Here's how the part is built. I have some questions about the finished solid (model axes, mm). Face numbers are marked on the shaded views. A direction names the side the tool comes from. Give positions to 0.01 mm unless a question says otherwise; leave off trailing zeros. Loops run counter-clockwise (first coordinate to the right, second up) from the corner with the lowest first, then second, coordinate; pieces in that order, holes last. Notation, with made-up numbers: (-17.5, -22) - (19.5, -22) arc R34 cw to (19.5, 15) - close; hole circle Ø6 at (-30.75, 48). An arc over 180 degrees is marked (long way). Use a Markdown table: item, result.
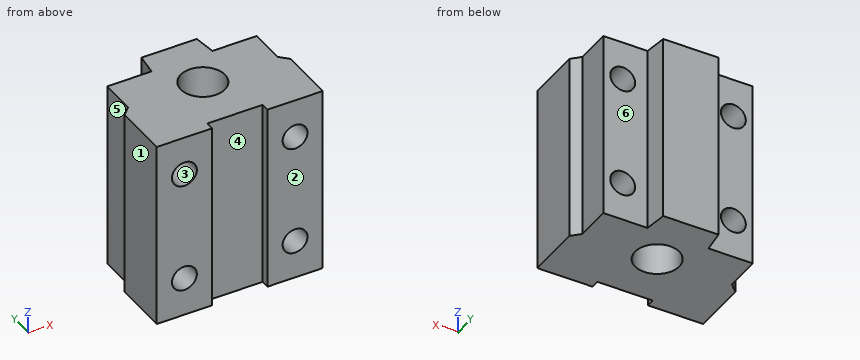
from build123d import *

# Parameters (mm, degrees)
SKETCH1_R           = 4
BOSS_EXTRUDE1_DEPTH = 34
SKETCH2_R           = 2.25
CUT_EXTRUDE1_DEPTH  = 42.291645644


with BuildPart() as part:
    # Sketch1 → Boss-Extrude1 (new body)
    with BuildSketch(Plane.XY):
        Polygon((5, -10), (-5, -10), (-5, -11.5), (-15, -11.5), (-15, -1.5), (-13.5, 0), (-13.5, 6.5), (-5.5, 6.5), (-5, 10.5), (5, 10.5), (5.5, 6.5), (13.5, 6.5), (13.5, 0), (15, -1.5), (15, -11.5), (5, -11.5), align=None)
        Circle(SKETCH1_R, mode=Mode.SUBTRACT)
    extrude(amount=BOSS_EXTRUDE1_DEPTH)

    # Sketch2 → Cut-Extrude1 (cut, through all)
    with BuildSketch(Plane(origin=(0, 6.5, 0), x_dir=(1, 0, 0), z_dir=(0, 1, 0))):
        with Locations(Location((10, -27, 0), (0, 0, 270))):
            Circle(SKETCH2_R)
        with Locations(Location((10, -7, 0), (0, 0, 270))):
            Circle(SKETCH2_R)
    cut_extrude1 = extrude(amount=-CUT_EXTRUDE1_DEPTH, mode=Mode.SUBTRACT)

    # Mirror1: Cut-Extrude1 across plane
    add(cut_extrude1.mirror(Plane(origin=(0, 0, 0), x_dir=(0, 0, 1), z_dir=(1, 0, 0))), mode=Mode.SUBTRACT)


solid = part.part
(1) Suppose I cut it at B-B on x = 0. Write out the boundary of the cut face in (y, z), plus the area to 3 significant figures.
A:
| item | result |
|---|---|
| outline | (-10, 0) - (-4, 0) - (-4, 34) - (-10, 34) - close; (4, 0) - (10.5, 0) - (10.5, 34) - (4, 34) - close |
| area | 425 mm2 |
(2) We'd pull the mould along X, two halves only. Please class the marked faces 1, 2 and 3: pulls with the +X half, pulls with the -X half, needs draft (parallel to the pull), parting line crosses it, or undercut.
A:
| item | result |
|---|---|
| face 1 | pulls with the -X half |
| face 2 | needs draft |
| face 3 | undercut |
(3) On a 3-axis mill with a long thin cutter (end or side, diameter ignored), from which of +Z, -Z, +X, -X, +Y, -Y can I reach the whole of each face in a straight line? I mean the marked faces 4, 5 and 6. Say none if no direction works.
A:
| item | result |
|---|---|
| face 4 | +Z, -Z, -Y |
| face 5 | +Z, -Z, -X, +Y |
| face 6 | +Z, -Z, +X, +Y |
(4) If I drill on line 1 (Z direction, x = -10, y = -3); line 2 (X direction, y = 0.25, z = 7); line 3 (X direction, y = -5.25, z = 27), over which ranges is the centre line in solid material (lowest first)?
A:
| item | result |
|---|---|
| line 1 | 0 to 4.75, 9.25 to 24.75, 29.25 to 34 |
| line 2 | -13.5 to -12.25, -7.75 to -3.99, 3.99 to 7.75, 12.25 to 13.5 |
| line 3 | -15 to -12.25, -7.75 to 7.75, 12.25 to 15 |
(5) Suppose I cut it at D-D on x = -10. Write out the boundary of the cut face in (y, z), plus the area to 3 significant figures.
A:
| item | result |
|---|---|
| outline | (-11.5, 0) - (6.5, 0) - (6.5, 4.75) - (-11.5, 4.75) - close; (-11.5, 9.25) - (6.5, 9.25) - (6.5, 24.75) - (-11.5, 24.75) - close; (-11.5, 29.25) - (6.5, 29.25) - (6.5, 34) - (-11.5, 34) - close |
| area | 450 mm2 |
(6) Suppose I cut it at C-C on y = 5.5. Write out the boundary of the cut face in (x, z).
A:
| item | result |
|---|---|
| outline | (-13.5, 0) - (13.5, 0) - (13.5, 34) - (-13.5, 34) - close; hole circle Ø4.5 at (-10, 7); hole circle Ø4.5 at (-10, 27); hole circle Ø4.5 at (10, 7); hole circle Ø4.5 at (10, 27) |
(7) Suppose I cut it at A-A on z = 7. Write out the boundary of the cut face in (x, y).
A:
| item | result |
|---|---|
| outline | (-15, -11.5) - (-12.25, -11.5) - (-12.25, 6.5) - (-13.5, 6.5) - (-13.5, 0) - (-15, -1.5) - close; (-7.75, -11.5) - (-5, -11.5) - (-5, -10) - (5, -10) - (5, -11.5) - (7.75, -11.5) - (7.75, 6.5) - (5.5, 6.5) - (5, 10.5) - (-5, 10.5) - (-5.5, 6.5) - (-7.75, 6.5) - close; (12.25, -11.5) - (15, -11.5) - (15, -1.5) - (13.5, 0) - (13.5, 6.5) - (12.25, 6.5) - close; hole circle Ø8 at (0, 0) |
(8) Will these pins go through, and if not, where does the flat tip stop? pin 1 (6 mm diameter, centred on x = 1.5, z = 6.5, fed in from -Y); pin 2 (5 mm diameter, centred on x = 10, z = 27, fed in from +Y); pin 3 (6.5 mm diameter, centred on x = 0, y = 0, fed in from +Z); pin 4 (10 mm diameter, centred on y = 0.5, z = 25, fed in from +X).
A:
| item | result |
|---|---|
| pin 1 | y = -10 |
| pin 2 | y = 6.5 |
| pin 3 | through |
| pin 4 | x = 15 |
